Verification items for the finished model (mm, model axes). A direction names the side the tool comes from. Round coordinates to 2 decimals unless told otherwise and drop trailing zeros. Write each loop counter-clockwise with the first axis right and the second up, starting at its lowest first coordinate (ties: lowest second). Pieces come first, ordered by that corner, then holes.
from build123d import *

# Parameters (mm, degrees)
BOSS_EXTRUDE1_DEPTH = 1.524
SKETCH2_W           = 15.1638
SKETCH2_H           = 12.1412
CUT_EXTRUDE1_DEPTH  = 22.375167739
BOSS_EXTRUDE2_DEPTH = 1.524
BOSS_EXTRUDE3_DEPTH = 0.6096
SKETCH7_W           = 15.24
SKETCH7_H           = 1.524
BOSS_EXTRUDE4_DEPTH = 0.508


with BuildPart() as part:
    # Sketch1 → Boss-Extrude1 (new body)
    with BuildSketch(Plane(origin=(0, 0, 0), x_dir=(1, 0, 0), z_dir=(0, 1, 0))):
        with BuildLine():
            Line((0, 0), (15.7988, 0))
            ThreePointArc((15.7988, 0), (16.696825612, 0.371974388), (17.0688, 1.27))
            Line((17.0688, 1.27), (17.0688, 11.5062))
            ThreePointArc((17.0688, 11.5062), (16.696825612, 12.404225612), (15.7988, 12.7762))
            Line((15.7988, 12.7762), (0, 12.7762))
            Line((0, 12.7762), (0, 0))
        make_face()
    extrude(amount=BOSS_EXTRUDE1_DEPTH)

    # Sketch2 → Cut-Extrude1 (cut, through all)
    with BuildSketch(Plane(origin=(0, 1.524, 0), x_dir=(1, 0, 0), z_dir=(0, 1, 0))):
        with Locations((8.6614, 6.3881)):
            Rectangle(SKETCH2_W, SKETCH2_H)
    extrude(amount=-CUT_EXTRUDE1_DEPTH, mode=Mode.SUBTRACT)

    # Sketch3 → Boss-Extrude2 (add)
    with BuildSketch(Plane(origin=(0, 0, 0), x_dir=(1, 0, 0), z_dir=(0, 1, 0))):
        Polygon((12.369415055, 0.3175), (16.2433, 4.191384945), (16.2433, 0.3175), align=None)
    extrude(amount=BOSS_EXTRUDE2_DEPTH)

    # Sketch5 → Boss-Extrude3 (add)
    with BuildSketch(Plane(origin=(0, 0, 0), x_dir=(1, 0, 0), z_dir=(0, 1, 0))):
        Polygon((1.0795, 0.3175), (12.369415055, 0.3175), (16.2433, 4.191384945), (16.2433, 12.4587), (1.0795, 12.4587), align=None)
        Polygon((1.7145, 11.8237), (1.7145, 0.9525), (12.106389443, 0.9525), (15.6083, 4.454410557), (15.6083, 11.8237), align=None, mode=Mode.SUBTRACT)
    extrude(amount=BOSS_EXTRUDE3_DEPTH)

    # Sketch7 → Boss-Extrude4 (add)
    with BuildSketch(Plane.ZY):
        with Locations((-6.3881, 0.762)):
            Rectangle(SKETCH7_W, SKETCH7_H)
    extrude(amount=BOSS_EXTRUDE4_DEPTH)


solid = part.part
Q1. Sectioned sample at B-B (y = 1). Enter the section's corners in (x, z).
Recorded:
outline: (-0.51, -14.01) - (0, -14.01) - (0, -12.78) - (15.8, -12.78) arc R1.27 ccw to (17.07, -11.51) - (17.07, -1.27) arc R1.27 ccw to (15.8, 0) - (0, 0) - (0, 1.23) - (-0.51, 1.23) - close; hole (1.08, -12.46) - (16.24, -12.46) - (16.24, -4.19) - (12.37, -0.32) - (1.08, -0.32) - close
Q2. Sectioned sample at D-D (x = 16). Enter the section's corners in (y, z).
Recorded:
outline: (0, -12.76) - (1.52, -12.76) - (1.52, -12.46) - (0.61, -12.46) - (0.61, -3.95) - (1.52, -3.95) - (1.52, -0.02) - (0, -0.02) - close
Q3. Release check for a two-part mould opening along Z. For faces 1 (the flat face through (0, 1, -13)), 2 (the flat face through (8, 1, -12.776)), 3 (the flat face through (8, 1, 0)), 4 (the flat face through (16.243, 1, -8)) record: released by +Z, released by -Z, zero draft, split by the parting line, or undercut.
Recorded:
face 1: zero draft
face 2: released by -Z
face 3: released by +Z
face 4: undercut
Q4. Sectioned sample at C-C (x = 9.5). Enter the section's corners in (y, z).
Recorded:
outline: (0, -12.78) - (1.52, -12.78) - (1.52, -12.46) - (0.61, -12.46) - (0.61, -11.82) - (0, -11.82) - close; (0, -0.95) - (0.61, -0.95) - (0.61, -0.32) - (1.52, -0.32) - (1.52, 0) - (0, 0) - close
Q5. Material ranges on line 1 along Z through (x, y) = (5.5, 0.2); line 2 along Z through (x, y) = (8.5, 0.65); line 3 along X through (y, z) = (0.1, -5), recorded low to high.
Recorded:
line 1: z = -12.78 to -11.82, -0.95 to 0
line 2: z = -12.78 to -12.46, -0.32 to 0
line 3: x = -0.51 to 1.71, 15.61 to 17.07
Q6. Sectioned sample at A-A (z = -7.25). Enter the section's corners in (x, y), plus the area to 3 significant figures.
Recorded:
outline: (-0.51, 0) - (1.71, 0) - (1.71, 0.61) - (1.08, 0.61) - (1.08, 1.52) - (-0.51, 1.52) - close; (15.61, 0) - (17.07, 0) - (17.07, 1.52) - (16.24, 1.52) - (16.24, 0.61) - (15.61, 0.61) - close
area: 4.45 mm2
Q7. Depth check by flat-ended pin: P1, Ø0.5, axis at x = 10, y = 1, coming from the +Z side; P2, Ø4, axis at x = 5, z = -9.5, coming from the +Y side. Enter the tip coordinate at first touch or a pass-through.
Recorded:
P1: stops at z = 0
P2: passes through
Q8. Tool access check on faces 5 (the cylindrical face through (16.7, 0.8, -12.4)), 6 (the flat face through (13.833, 0.301, -2.679)), 7 (the flat face through (17.069, 1, -6)), 8 (the flat face through (0, 1, 1)), 9 (the flat face through (7, 1, -0.317)). Record the directions out of +Z, -Z, +X, -X, +Y, -Y that give a thin tool (end or side, any length) a straight path to the whole face; none if there is none.
Recorded:
face 5: -Z, +X, +Y, -Y
face 6: +Y, -Y
face 7: +Z, -Z, +X, +Y, -Y
face 8: +Z, +X, +Y, -Y
face 9: +Y
